```python
from build123d import *

# Parameters (mm, degrees)
CROQUIS1_R              = 11
SALIENTE_EXTRUIR1_DEPTH = 5
CROQUIS2_R              = 4.8
SALIENTE_EXTRUIR2_DEPTH = 5
CROQUIS3_R              = 1.6
CORTAR_EXTRUIR1_DEPTH   = 6
CROQUIS4_R              = 3.575
CORTAR_EXTRUIR2_DEPTH   = 11
CROQUIS5_R              = 3.25
CORTAR_EXTRUIR3_DEPTH   = 3.5


with BuildPart() as part:
    # Croquis1 → Saliente-Extruir1 (new body)
    with BuildSketch(Plane(origin=(0, 0, 0), x_dir=(1, 0, 0), z_dir=(0, 1, 0))):
        Circle(CROQUIS1_R)
    extrude(amount=SALIENTE_EXTRUIR1_DEPTH)

    # Croquis2 → Saliente-Extruir2 (add)
    with BuildSketch(Plane.XZ):
        Circle(CROQUIS2_R)
    extrude(amount=SALIENTE_EXTRUIR2_DEPTH)

    # Croquis3 → Cortar-Extruir1 (cut, through all)
    with BuildSketch(Plane.XZ):
        with Locations((-7.9, 0)):
            Circle(CROQUIS3_R)
        with Locations((7.9, 0)):
            Circle(CROQUIS3_R)
    extrude(amount=-CORTAR_EXTRUIR1_DEPTH, mode=Mode.SUBTRACT)

    # Croquis4 → Cortar-Extruir2 (cut, through all)
    with BuildSketch(Plane.XZ.offset(5)):
        Circle(CROQUIS4_R)
    extrude(amount=-CORTAR_EXTRUIR2_DEPTH, mode=Mode.SUBTRACT)

    # Croquis5 → Cortar-Extruir3 (cut)
    with BuildSketch(Plane(origin=(0, 5, 0), x_dir=(1, 0, 0), z_dir=(0, 1, 0))):
        with Locations((-7.9, 0)):
            Circle(CROQUIS5_R)
        with Locations((7.9, 0)):
            Circle(CROQUIS5_R)
    extrude(amount=-CORTAR_EXTRUIR3_DEPTH, mode=Mode.SUBTRACT)


solid = part.part
```
Verification items for the finished model (mm, model axes). A direction names the side the tool comes from. Give positions to 0.01 mm unless a question says otherwise; leave off trailing zeros. Order: outer loops, then holes, each group sorted by start corner. A loop starts at its lowest first (then second) coordinate and runs counter-clockwise, first axis right, second up. Notation, with made-up numbers: M 54.25,77.25 L 81.25,77.25 A5 cw 81.25,81.25 Z; hole C 42,55 d2. An arc over 180 degrees is marked long. Return JSON: item names as keys, results as strings. Group by question number.
1) Access from +Z, -Z, +X, -X, +Y, -Y to the whole of each face (thin tool, end or side, straight path). Record for faces 1 (the face through (-4.652, 3.274, 0.126)), 2 (the face through (9.426, 0.74, 0.481)).
2) Section check B-B on x = -4.25. Record the cut outline in (y, z), and give its area (3 significant figures).
3) Scan lines: line 1 (Y direction, x = 4, z = -7.5); line 2 (Z direction, x = -9, y = 0.75); line 3 (Z direction, x = 0.5, y = -4.5). Record each from-to range of solid material in increasing order.
4) Mould release check, pull along X, two halves, no side actions. Record for faces 3 (the face through (-9.5, 0.74, 0.07)), 4 (the face through (2.58, -2.46, 4.05)), 5 (the face through (2, 0, 5)): pulls with the +X half, pulls with the -X half, needs draft (parallel to the pull), parting line crosses it, or undercut.
5) Go/stop test with flat-tipped pins: pin 1 Ø4 at (x, z) = (-7.9, 0) entering from -Y; pin 2 Ø5 at (x, z) = (-8, -0.5) entering from +Y; pin 3 Ø3 at (x, y) = (-4, -4) entering from +Z; pin 4 Ø3 at (x, z) = (7.9, 0) entering from +Y. Record where each tip stops, or that it passes through.
6) Section check A-A on x = 0. Record the cut outline in (y, z) (3 decimals), and give its area (3 significant figures).
7) Section check C-C on y = 3.25. Record the cut outline in (x, z) (3 decimals), and give its area (3 significant figures).
8) Section check D-D on z = 4. Record the cut outline in (x, y), and give its area (3 significant figures).
Answer block:
{
 "1": {"face 1": "+Y", "face 2": "+Y, -Y"},
 "2": {"outline": "M -5,-2.23 L 0,-2.23 L 0,-10.15 L 5,-10.15 L 5,10.15 L 0,10.15 L 0,2.23 L -5,2.23 Z", "area": "124 mm^2"},
 "3": {"line 1": "y = 0 to 5", "line 2": "z = -6.32 to -1.16, 1.16 to 6.32", "line 3": "z = -4.77 to -3.54, 3.54 to 4.77"},
 "4": {"face 3": "undercut", "face 4": "parting line crosses it", "face 5": "needs draft"},
 "5": {"pin 1": "stops at y = 0", "pin 2": "stops at y = 1.5", "pin 3": "stops at z = 4.1", "pin 4": "passes through"},
 "6": {"outline": "M -5,-4.8 L 0,-4.8 L 0,-11 L 5,-11 L 5,-3.575 L -5,-3.575 Z; M -5,3.575 L 5,3.575 L 5,11 L 0,11 L 0,4.8 L -5,4.8 Z", "area": "86.5 mm^2"},
 "7": {"outline": "M -10.94,-1.15 A11 ccw 10.94,-1.15 A3.25 cw long 10.94,1.15 A11 ccw -10.94,1.15 A3.25 cw long Z; hole C 0,0 d7.15", "area": "274 mm^2"},
 "8": {"outline": "M -10.25,0 L -2.65,0 L -2.65,-5 L 2.65,-5 L 2.65,0 L 10.25,0 L 10.25,5 L -10.25,5 Z", "area": "129 mm^2"}
}
